Part model, mm, in its own coordinate system. A direction names the side the tool comes from. Round coordinates to 2 decimals unless told otherwise and drop trailing zeros. Write each loop counter-clockwise with the first axis right and the second up, starting at its lowest first coordinate (ties: lowest second). Pieces come first, ordered by that corner, then holes. Notation, with made-up numbers: (37, 18) -> (79, 18) arc R7 cw to (79, 31) -> close; hole circle Ø11 at (2.25, -12). An arc over 180 degrees is marked (long way). Return JSON: item names as keys, results as strings. Group by question number.
(1) Saw through at B-B (y = 0). List the corners of the cut face in (x, z).
(2) Tool access for faces 1 (the flat face through (-11, 11.35, 2)), 2 (the cylindrical face through (-26.349, -4.868, 5.972)), 3 (the flat face through (6.1, -5, 2)): list every direction of +Z, -Z, +X, -X, +Y, -Y with a clear straight run to the whole face (end or side of a thin tool).
(3) Saw through at D-D (y = 8.9). List the corners of the cut face in (x, z).
(4) Drop flat-ended pins along their axis: pin 1 Ø1.5 at (y, z) = (6.5, 5) entering from +X; pin 2 Ø2 at (x, y) = (0, -19.2) entering from +Z. Give the stop position or say it passes through.
(5) Mould opens along Y. For faces 4 (the flat face through (-11, -5, 0)), 5 (the cylindrical face through (-24.496, 0.198, 1.479)), 6 (the flat face through (-11, -21.65, 2)) say: +Y half, -Y half, draft (parallel to the pull), parting line (faces both ways), or undercut.
(6) Saw through at C-C (z = 2). List the corners of the cut face in (x, y).
(7) Saw through at A-A (x = 2). List the corners of the cut face in (y, z).
(8) Drill centre lines: L1, parallel to X at y = 0, z = 1.4; L2, parallel to Y at x = 0, z = 1.1; L3, parallel to Y at x = -20, z = 1.95. Where is each one in solid material? Low to high. Write a range as from..to.
from build123d import *

# Parameters (mm, degrees)
SKETCH1_W           = 39.1
SKETCH1_H           = 33
SKETCH1_R           = 0.95
SKETCH1_R_2         = 4.5
SKETCH1_W_2         = 12.2
SKETCH1_H_2         = 22.7
BOSS_EXTRUDE1_DEPTH = 4
BOSS_EXTRUDE2_START = 4
SKETCH2_R           = 8
SKETCH2_R_2         = 4.403773093
BOSS_EXTRUDE2_DEPTH = 4
CUT_EXTRUDE1_START  = 8
SKETCH3_R           = 5.6
CUT_EXTRUDE1_DEPTH  = 5


with BuildPart() as part:
    # Sketch1 → Boss-Extrude1 (new body)
    with BuildSketch(Plane.XY):
        with Locations((-10.45, -5.15)):
            Rectangle(SKETCH1_W, SKETCH1_H)
        with Locations((0, 8.9)):
            Circle(SKETCH1_R, mode=Mode.SUBTRACT)
        with Locations((0, -19.2)):
            Circle(SKETCH1_R, mode=Mode.SUBTRACT)
        with Locations((-20, 0)):
            Circle(SKETCH1_R_2, mode=Mode.SUBTRACT)
        with Locations((0, -5.15)):
            Rectangle(SKETCH1_W_2, SKETCH1_H_2, mode=Mode.SUBTRACT)
    extrude(amount=BOSS_EXTRUDE1_DEPTH)

    # Sketch2 → Boss-Extrude2 (add)
    with BuildSketch(Plane.XY.offset(BOSS_EXTRUDE2_START)):
        with Locations((-20, 0)):
            Circle(SKETCH2_R)
        with Locations((-20, 0)):
            Circle(SKETCH2_R_2, mode=Mode.SUBTRACT)
    extrude(amount=BOSS_EXTRUDE2_DEPTH)

    # Sketch3 → Cut-Extrude1 (cut)
    with BuildSketch(Plane.XY.offset(CUT_EXTRUDE1_START)):
        with Locations((-20, 0)):
            Circle(SKETCH3_R)
    extrude(amount=-CUT_EXTRUDE1_DEPTH, mode=Mode.SUBTRACT)


solid = part.part
Computed values:
{
 "1": {"outline": "(-30, 0) -> (-24.5, 0) -> (-24.5, 3) -> (-25.6, 3) -> (-25.6, 8) -> (-28, 8) -> (-28, 4) -> (-30, 4) -> close; (-15.5, 0) -> (-6.1, 0) -> (-6.1, 4) -> (-12, 4) -> (-12, 8) -> (-14.4, 8) -> (-14.4, 3) -> (-15.5, 3) -> close; (6.1, 0) -> (9.1, 0) -> (9.1, 4) -> (6.1, 4) -> close"},
 "2": {"face 1": "+Z, -Z, +X, -X, +Y", "face 2": "+Z", "face 3": "+Z, -Z"},
 "3": {"outline": "(-30, 0) -> (-0.95, 0) -> (-0.95, 4) -> (-30, 4) -> close; (0.95, 0) -> (9.1, 0) -> (9.1, 4) -> (0.95, 4) -> close"},
 "4": {"pin 1": "x = -14.44", "pin 2": "z = 4"},
 "5": {"face 4": "draft", "face 5": "undercut", "face 6": "-Y half"},
 "6": {"outline": "(-30, -21.65) -> (9.1, -21.65) -> (9.1, 11.35) -> (-30, 11.35) -> close; hole circle Ø9 at (-20, 0); hole (-6.1, -16.5) -> (6.1, -16.5) -> (6.1, 6.2) -> (-6.1, 6.2) -> close; hole circle Ø1.9 at (0, -19.2); hole circle Ø1.9 at (0, 8.9)"},
 "7": {"outline": "(-21.65, 0) -> (-16.5, 0) -> (-16.5, 4) -> (-21.65, 4) -> close; (6.2, 0) -> (11.35, 0) -> (11.35, 4) -> (6.2, 4) -> close"},
 "8": {"L1": "-30..-24.5, -15.5..-6.1, 6.1..9.1", "L2": "-21.65..-20.15, -18.25..-16.5, 6.2..7.95, 9.85..11.35", "L3": "-21.65..-4.5, 4.5..11.35"}
}
